Autodesk Inventor part; units mm, degrees
ref_plane "Right" through (0, 0, 0) normal (1, 0, 0) x (0, 1, 0)
ref_plane "Top" through (0, 0, 0) normal (0, 1, 0) x (-1, 0, 0)
ref_plane "Front" through (0, 0, 0) normal (0, 0, 1) x (1, 0, 0)
sketch "Sketch1" plane through (0, 0, 0) normal (1, 0, 0) x (0, 1, 0)
  line L0 (-40, 15) -> (40, 15)
  line L1 (40, 15) -> (40, -15)
  line L2 (40, -15) -> (-40, -15)
  line L3 (-40, -15) -> (-40, 15)
  line L4 (-40, 15) -> (40, -15) construction
  line L5 (40, 15) -> (-40, -15) construction
  point P0 (0, 0)
  dimension "d0" = 30
  dimension "d1" = 80
extrude "Extrusion1" add sketch "Sketch1" along normal mid plane 140.5
sketch "Sketch2" plane through (-70.25, -40, 15) normal (0, 0, 1) x (1, 0, 0)
  line L0 (140.5, 80) -> (0, 80) construction
  line L1 (0, 0) -> (0, 80) construction
  line L2 (0, 80) -> (0, 58.75)
  line L3 (0, 58.75) -> (34, 80)
  line L4 (34, 80) -> (0, 80)
  line L5 (0, 21.25) -> (0, 0)
  line L6 (0, 0) -> (34, 0)
  line L7 (34, 0) -> (0, 21.25)
  point P0 (70.25, 40)
  dimension "d4" = 37.5
  dimension "d5" = 106.5
  dimension "d6" = 147.995
extrude "Extrusion2" cut sketch "Sketch2" against normal through all
sketch "Sketch3" plane through (70.25, -40, 15) normal (0, 0, 1) x (1, 0, 0)
  line L0 (0, 80) -> (0, 0) construction
  line L1 (-140.5, 21.25) -> (-140.5, 58.75) construction
  line L2 (-140.5, 57.1) -> (0, 57.1)
  line L3 (0, 57.1) -> (0, 22.9)
  line L4 (0, 22.9) -> (-140.5, 22.9)
  line L5 (-140.5, 22.9) -> (-140.5, 57.1)
  point P0 (-70.25, 40)
  point P1 (-140.5, 40)
  dimension "d9" = 34.2
extrude "Extrusion3" cut sketch "Sketch3" against normal blind 2
sketch "Sketch4" plane through (-36.25, 40, 15) normal (0, 0, 1) x (1, 0, 0)
  line L0 (106.5, -57.1) -> (-34, -57.1) construction
  line L1 (-34, -58.75) -> (-34, -57.1) construction
  line L2 (-34, -58.75) -> (0, -80) construction
  line L3 (0, -80) -> (106.5, -80) construction
  line L4 (106.5, -57.1) -> (106.5, -80) construction
  line L5 (-34, -22.9) -> (106.5, -22.9) construction
  line L6 (-34, -57.1) -> (-34, -22.9) construction
  line L7 (106.5, -57.1) -> (-34, -57.1) construction
  line L8 (106.5, -22.9) -> (106.5, -57.1) construction
  line L9 (106.5, -22) -> (80.5, -22)
  line L10 (80.5, -22) -> (80.5, -58)
  line L11 (80.5, -58) -> (106.5, -58)
  line L12 (106.5, -58) -> (106.5, -22)
  line L13 (85.625, -21.875) -> (85.625, -58.125) construction
  line L14 (90.75, -21.875) -> (90.75, -58.125)
  line L15 (80.5, -58.125) -> (80.5, -21.875)
  arc A0 (90.75, -21.875) -> (80.5, -21.875) centre (85.625, -21.875) ccw
  arc A1 (80.5, -58.125) -> (90.75, -58.125) centre (85.625, -58.125) ccw
  point P0 (36.25, -40)
  point P1 (106.5, -40)
  point P2 (85.625, -40)
  point P3 (80.5, -40)
  dimension "d12" = 36
  dimension "d13" = 26
  dimension "d14" = 46.5
  dimension "d15" = 15.75
extrude "Extrusion4" cut sketch "Sketch4" against normal blind 9.5
sketch "Sketch5" plane through (70.25, -40, 13) normal (0, 0, 1) x (1, 0, 0)
  line L0 (-26, 22.9) -> (-26, 57.1) construction
  line L1 (-15.75, 58) -> (0, 58) construction
  line L2 (-15.75, 58.125) -> (-15.75, 58) construction
  arc A0 (-15.75, 58.125) -> (-26, 58.125) centre (-20.875, 58.125) ccw construction
  line L3 (-26, 21.875) -> (-26, 58.125) construction
  arc A1 (-26, 21.875) -> (-15.75, 21.875) centre (-20.875, 21.875) ccw construction
  line L4 (-15.75, 22) -> (-15.75, 21.875) construction
  line L5 (0, 22) -> (-15.75, 22) construction
  line L6 (0, 58) -> (0, 22) construction
  line L7 (-90.5, 40) -> (-50.5, 40)
  circle A2 centre (-90.5, 40) radius 4.25
  circle A3 centre (-50.5, 40) radius 4.25
  point P0 (-70.25, 40)
  dimension "d18" = 8.5
  dimension "d19" = 48.5
  dimension "d20" = 20.25
  dimension "d23" = 50.5
  dimension "d24" = 40
hole "Hole1" at (-20.25, 0, 13) at (19.75, 0, 13) direction (0, 0, -1) diameter 8.509 end through all
equation "\"BendRadius\" = Thickness"
equation "\"BendReliefWidth\" = 0.5 * Thickness"
equation "\"BendReliefDepth\" = 0.5 * Thickness"
equation "\"CornerReliefSize\" = 4 * Thickness"
equation "\"MinimumRemnant\" = 2 * Thickness"
equation "\"TransitionRadius\" = BendRadius"
equation "\"JacobiRadiusSize\" = BendRadius"
properties part number "DHC-1500-FF-02-002" material "A36"
Model file for the job. Use its own axes, mm. A direction names the side the tool comes from. Coordinates: 2 decimals unless noted, no trailing zeros. Write each loop counter-clockwise with the first axis right and the second up, starting at its lowest first coordinate (ties: lowest second). Pieces come first, ordered by that corner, then holes. Notation, with made-up numbers: (12.5, 70) -> (43.5, 70) arc R13 ccw to (43.5, 82) -> close; hole circle Ø4 at (43, 74). An arc over 180 degrees is marked (long way). One line per item, written item: value. Start each with the question number.
1) Slice it at A-A on x = -20.25. Write the cut outline in (y, z).
2) Which spindle directions (+Z, -Z, +X, -X, +Y, -Y) get a long thin tool onto all of the face, cutting with end or side? Do faces 4 (the face through (62, 18, 10)), 5 (the face through (23.903, 0.922, -1.196)), 6 (the face through (49.49, 23.25, 10.32)). Say none if no direction does.
3) Probe probe 1 along X at (y, z) = (0, 4.5); probe 2 along Y at (x, z) = (19.75, -8.75); probe 3 along X at (y, z) = (2, -11.75). List the from-to ranges inside material, lowest first.
4) Slice it at C-C on z = -11.75. Write the cut outline in (x, y).
5) Slice it at D-D on y = 9.5. Write the cut outline in (x, z).
6) Slice it at B-B on y = 0. Write the cut outline in (x, z).
7) Pull direction Y, two halves, no side cores. Call faces 1 (the face through (16, 40, 0)), 2 (the face through (-1, 28, 15)), 3 (the face through (-14, 0, 13)): +Y half, -Y half, draft (parallel to the pull), parting line (faces both ways), or undercut.
8) Flat gauge pins, fed straight in: pin 1 Ø10.5 at (y, z) = (2.5, 12.5) entering from +X; pin 2 Ø10.5 at (x, y) = (-18.5, 5) entering from +Z; pin 3 Ø13 at (x, y) = (56.5, 1.5) entering from +Z. Where does each tip first touch, or does it go through?
Answers follow:
1. outline: (-40, -15) -> (-4.25, -15) -> (-4.25, 13) -> (-17.1, 13) -> (-17.1, 15) -> (-40, 15) -> close; (4.25, -15) -> (40, -15) -> (40, 15) -> (17.1, 15) -> (17.1, 13) -> (4.25, 13) -> close
2. face 4: +Z, +X
2. face 5: +Z, -Z
2. face 6: +Z
3. probe 1: -70.25 to -24.5, -16 to 15.5, 24 to 70.25
3. probe 2: -40 to -4.25, 4.25 to 40
3. probe 3: -70.25 to -24.01, -16.49 to 15.99, 23.51 to 70.25
4. outline: (-70.25, -18.75) -> (-36.25, -40) -> (70.25, -40) -> (70.25, 40) -> (-36.25, 40) -> (-70.25, 18.75) -> close; hole circle Ø8.51 at (-20.25, 0); hole circle Ø8.51 at (19.75, 0)
5. outline: (-70.25, -15) -> (70.25, -15) -> (70.25, 5.5) -> (44.25, 5.5) -> (44.25, 13) -> (-70.25, 13) -> close
6. outline: (-70.25, -15) -> (-24.5, -15) -> (-24.5, 13) -> (-70.25, 13) -> close; (-16, -15) -> (15.5, -15) -> (15.5, 13) -> (-16, 13) -> close; (24, -15) -> (70.25, -15) -> (70.25, 5.5) -> (44.25, 5.5) -> (44.25, 13) -> (24, 13) -> close
7. face 1: +Y half
7. face 2: draft
7. face 3: undercut
8. pin 1: x = 44.25
8. pin 2: z = 13
8. pin 3: z = 5.5
